Can you work these out from the model? Positions are in its coordinate system, mm. A direction names the side the tool comes from. Round coordinates to 2 decimals unless told otherwise and drop trailing zeros. Write each loop counter-clockwise with the first axis right and the second up, starting at its lowest first coordinate (ties: lowest second). Pieces come first, ordered by that corner, then holes. Notation, with made-up numbers: (53, 53.5) - (104, 53.5) arc R29 ccw to (104, 75.5) - close; hole circle Ø3 at (10, 82.5). An arc over 180 degrees is marked (long way). One line per item, written item: value. Start each with the question number.
(1) On a 3-axis mill with a long thin cutter (end or side, diameter ignored), from which of +Z, -Z, +X, -X, +Y, -Y can I reach the whole of each face in a straight line? I mean faces 4 (the face through (254, 13, 3.175)), 5 (the face through (254, 25.4, 20)). Say none if no direction works.
(2) I'm going to push flat-ended pins straight in: pin 1 Ø0.7 at (y, z) = (9, 2.5) entering from +X; pin 2 Ø4 at (x, z) = (502.72, 20) entering from -Y (1 decimal); pin 3 Ø6 at (x, y) = (317, 19.5) entering from -Z; pin 4 Ø1.1 at (y, z) = (9, 37) entering from -X. Where does each tip first touch, or does it pass through?
(3) I want a section at B-B on x = 134.5. List the corners of the cut face in (y, z) for me (3 decimals), plus the area to 3 significant figures.
(4) I want a section at A-A on y = 14. List the corners of the cut face in (x, z) for me (1 decimal).
(5) Thinking about a two-plate mould opening in Z: for faces 1 (the face through (261.3, 22.225, 19.7)), 2 (the face through (487.31, 12.52, 0.67)), 3 (the face through (254, 0, 20)), which applies, +Z half, -Z half, draft (parallel to the pull), parting line (faces both ways), or undercut?
(6) I want a section at C-C on z = 28.5. List the corners of the cut face in (x, y) for me (3 decimals), plus the area to 3 significant figures.
(7) If I drill on L1, parallel to Z at x = 369.5, y = 19 (3 decimals); L2, parallel to Y at x = 305, z = 33.5 (3 decimals); L3, parallel to Z at x = 12.78, y = 2.1 (3 decimals), over which ranges is the centre line in solid material (lowest first)? Write a range as from..to.
from build123d import *

# Parameters (mm, degrees)
SKETCH1_W           = 515.5
SKETCH1_H           = 40
SKETCH1_R           = 3.175
BOSS_EXTRUDE1_DEPTH = 25.4
CUT_EXTRUDE1_REACH  = 519.673
SKETCH2_W           = 33.65
SKETCH2_H           = 19.05
SKETCH4_W           = 40
SKETCH4_H           = 19.05
CUT_EXTRUDE2_DEPTH  = 24
FILLET1_R           = 35


with BuildPart() as part:
    # Sketch1 → Boss-Extrude1 (new body)
    with BuildSketch(Plane(origin=(0, 0, 0), x_dir=(1, 0, 0), z_dir=(0, 1, 0))):
        with Locations((257.75, -20)):
            Rectangle(SKETCH1_W, SKETCH1_H)
        with Locations(Location((257.75, -20, 0), (0, 0, 270))):
            Circle(SKETCH1_R, mode=Mode.SUBTRACT)
        with Locations(Location((12.78, -20, 0), (0, 0, 270))):
            Circle(SKETCH1_R, mode=Mode.SUBTRACT)
        with Locations(Location((502.72, -20, 0), (0, 0, 90))):
            Circle(SKETCH1_R, mode=Mode.SUBTRACT)
    extrude(amount=BOSS_EXTRUDE1_DEPTH)

    # Cut-Extrude1: up to this face of the body (flat: up to its plane)
    cut_extrude1_end = Plane(part.part.faces().sort_by_distance((515.5, 12.7, 20))[0])
    # Sketch2 → Cut-Extrude1 (cut, up to the picked face)
    with BuildSketch(Plane.ZY, mode=Mode.PRIVATE) as cut_extrude1_sk1:
        with Locations((20, 12.7)):
            Rectangle(SKETCH2_W, SKETCH2_H)
    cut_extrude1_tool1 = split(extrude(cut_extrude1_sk1.sketch, amount=-CUT_EXTRUDE1_REACH, mode=Mode.PRIVATE), bisect_by=cut_extrude1_end, keep=Keep.BOTH, mode=Mode.PRIVATE)
    add(cut_extrude1_tool1.solids().sort_by(Axis((0, 12.7, 20), (1, 0, 0)))[0], mode=Mode.SUBTRACT)

    # Sketch4 → Cut-Extrude2 (cut)
    with BuildSketch(Plane.ZY):
        with Locations((20, 12.7)):
            Rectangle(SKETCH4_W, SKETCH4_H)
    cut_extrude2 = extrude(amount=-CUT_EXTRUDE2_DEPTH, mode=Mode.SUBTRACT)

    # Mirror1: Cut-Extrude2 across plane
    add(cut_extrude2.mirror(Plane.ZY.offset(-257.75)), mode=Mode.SUBTRACT)

    # Fillet1
    # the kernel refuses this fillet: 35 mm, written as the material it takes off along each edge
    with BuildSketch(Plane(origin=(515.5, -65.275, 0), x_dir=(-1, 0, 0), z_dir=(0, 1, 0)), Plane(origin=(0, -65.275, 40), x_dir=(1, 0, 0), z_dir=(0, 1, 0))) as fillet1_piece_1:
        with BuildLine():
            CenterArc((FILLET1_R, FILLET1_R), FILLET1_R, 180, 90)
            Line((0, FILLET1_R), (0, 0))
            Line((0, 0), (FILLET1_R, 0))
        make_face()
    extrude(amount=178.175, mode=Mode.SUBTRACT)
    with BuildSketch(Plane(origin=(515.5, -65.275, 40), x_dir=(-1, 0, 0), z_dir=(0, 1, 0)), Plane(origin=(0, -65.275, 0), x_dir=(1, 0, 0), z_dir=(0, 1, 0))) as fillet1_piece_2:
        with BuildLine():
            CenterArc((FILLET1_R, -FILLET1_R), FILLET1_R, 90, 90)
            Line((0, -FILLET1_R), (0, 0))
            Line((0, 0), (FILLET1_R, 0))
        make_face()
    extrude(amount=178.175, mode=Mode.SUBTRACT)


solid = part.part
Established:
1. face 4: +X, -X
1. face 5: +Z, -Z, +X, -X, +Y
2. pin 1: x = 491.5
2. pin 2: through
2. pin 3: z = 0
2. pin 4: x = 24
3. outline: (0, 0) - (25.4, 0) - (25.4, 40) - (0, 40) - close; hole (3.175, 3.175) - (22.225, 3.175) - (22.225, 36.825) - (3.175, 36.825) - close
3. area: 375 mm2
4. outline: (24, 1.8) arc R35 ccw to (35, 0) - (480.5, 0) arc R35 ccw to (491.5, 1.8) - (491.5, 3.2) - (24, 3.2) - close; (24, 36.8) - (491.5, 36.8) - (491.5, 38.2) arc R35 ccw to (480.5, 40) - (35, 40) arc R35 ccw to (24, 38.2) - close
5. face 1: undercut
5. face 2: -Z half
5. face 3: draft
6. outline: (9.063, 0) - (506.437, 0) - (506.437, 3.175) - (9.063, 3.175) - close; (9.063, 22.225) - (506.437, 22.225) - (506.437, 25.4) - (9.063, 25.4) - close
6. area: 3,160 mm2
7. L1: 0..3.175, 36.825..40
7. L2: 0..3.175, 22.225..25.4
7. L3: 7.958..16.825, 23.175..32.042
